Geometry check sheet. Reference: the model listing, model coordinates, mm. A direction names the side the tool comes from. Give positions to 0.01 mm unless a question says otherwise; leave off trailing zeros. Order: outer loops, then holes, each group sorted by start corner. A loop starts at its lowest first (then second) coordinate and runs counter-clockwise, first axis right, second up. Notation, with made-up numbers: M 76,-11.5 L 129,-11.5 A7 cw 129,-6.5 Z; hole C 85,11 d8. An arc over 180 degrees is marked long. Answer as CSV lines item,"result". Start each with the question number.
```python
from build123d import *

# Parameters (mm, degrees)
F0_R     = 6.35
F1_DEPTH = 16.002
F2_DEPTH = 16.002
F3_R     = 9.652
F4_W     = 56.33977
F4_H     = 23.11277
F5_DEPTH = 16.002
F7_R     = 9.652
F8_DEPTH = 16.003


with BuildPart() as f1:
    # F0 (on Front) → F1 (new body)
    with BuildSketch(Plane.XZ):
        with BuildLine():
            Line((-50.8, 0), (0, 0))
            Line((0, 0), (50.8, 0))
            Line((50.8, 0), (50.8, 44.45))
            ThreePointArc((50.8, 44.45), (47.080256, 53.430256), (38.1, 57.15))
            ThreePointArc((38.1, 57.15), (29.119744, 53.430256), (25.4, 44.45))
            Line((25.4, 44.45), (25.4, 16.002))
            Line((25.4, 16.002), (0, 16.002))
            Line((0, 16.002), (-25.4, 16.002))
            Line((-25.4, 16.002), (-25.4, 44.45))
            ThreePointArc((-25.4, 44.45), (-29.119744, 53.430256), (-38.1, 57.15))
            ThreePointArc((-38.1, 57.15), (-47.080256, 53.430256), (-50.8, 44.45))
            Line((-50.8, 44.45), (-50.8, 0))
        make_face()
        with Locations((-38.1, 44.45)):
            Circle(F0_R, mode=Mode.SUBTRACT)
        with Locations((38.1, 44.45)):
            Circle(F0_R, mode=Mode.SUBTRACT)
    extrude(amount=F1_DEPTH)

    # F0 (on Front) → F2 (join)
    with BuildSketch(Plane.XZ):
        with BuildLine():
            Line((-50.8, 0), (0, 0))
            Line((0, 0), (50.8, 0))
            Line((50.8, 0), (50.8, 44.45))
            ThreePointArc((50.8, 44.45), (47.080256, 53.430256), (38.1, 57.15))
            ThreePointArc((38.1, 57.15), (29.119744, 53.430256), (25.4, 44.45))
            Line((25.4, 44.45), (25.4, 16.002))
            Line((25.4, 16.002), (0, 16.002))
            Line((0, 16.002), (-25.4, 16.002))
            Line((-25.4, 16.002), (-25.4, 44.45))
            ThreePointArc((-25.4, 44.45), (-29.119744, 53.430256), (-38.1, 57.15))
            ThreePointArc((-38.1, 57.15), (-47.080256, 53.430256), (-50.8, 44.45))
            Line((-50.8, 44.45), (-50.8, 0))
        make_face()
        with Locations((-38.1, 44.45)):
            Circle(F0_R, mode=Mode.SUBTRACT)
        with Locations((38.1, 44.45)):
            Circle(F0_R, mode=Mode.SUBTRACT)
    extrude(amount=F2_DEPTH)

    # F3
    f3_edges = [f1.edges().sort_by_distance(p)[0] for p in [
        (-25.4, -8.001, 16.002),
        (25.4, -8.001, 16.002),
    ]]
    fillet(f3_edges, radius=F3_R)

    # F4 (on Top) → F5 (join)
    with BuildSketch(Plane.XY):
        with Locations((0, -27.554179)):
            Rectangle(F4_W, F4_H)
    extrude(amount=F5_DEPTH)

    # F7
    f7_edges = [f1.edges().sort_by_distance(p)[0] for p in [
        (28.169885, -39.110564, 8.001),
        (-28.169885, -39.110564, 8.001),
        (28.169885, -16.002, 8.001),
        (-28.169885, -16.002, 8.001),
    ]]
    fillet(f7_edges, radius=F7_R)

    # F6 (on face) → F8 (cut, through all)
    with BuildSketch(Plane.XY.offset(16.002)):
        with BuildLine():
            Line((19.05, -21.026887), (0, -21.026887))
            Line((0, -21.026887), (-19.05, -21.026887))
            ThreePointArc((-19.05, -21.026887), (-25.4, -27.376887), (-19.05, -33.726887))
            Line((-19.05, -33.726887), (0, -33.726887))
            Line((0, -33.726887), (19.05, -33.726887))
            ThreePointArc((19.05, -33.726887), (25.4, -27.376887), (19.05, -21.026887))
        make_face()
    extrude(amount=-F8_DEPTH, mode=Mode.SUBTRACT)


solid = f1.part
```
Item 1: Depth check by flat-ended pin: pin 1 Ø10.5 at (x, z) = (-27.5, 23.5) entering from -Y; pin 2 Ø5 at (y, z) = (-19.5, 16.5) entering from -X; pin 3 Ø4 at (y, z) = (-27.5, 11.5) entering from -X. Enter the tip coordinate at first touch or a pass-through.
Item 2: Draft check along X on faces 1 (the face through (0, -39.111, 8)), 2 (the face through (-1, -19, 16.002)), 3 (the face through (-30.922, -18.904, 7.889)). Enter one of: pulls with the +X half, pulls with the -X half, needs draft (parallel to the pull), parting line crosses it, or undercut.
Item 3: Section check A-A on z = 32. Record the boundary of the cut face in (x, y), then the cut area to 3 significant figures.
Item 4: Section check B-B on y = -9.5. Record the boundary of the cut face in (x, z).
Item 5: Scan lines: line 1 along X through (y, z) = (-9, 44); line 2 along Z through (x, y) = (38, -3); line 3 along X through (y, z) = (-1.5, 48.5). Record each from-to range of solid material in increasing order.
Item 6: Section check D-D on z = 49.5. Record the boundary of the cut face in (x, y).
Item 7: Access from +Z, -Z, +X, -X, +Y, -Y to the whole of each face (thin tool, end or side, straight path). Record for faces 4 (the face through (41, -16.002, 29)), 5 (the face through (25.4, -27.5, 8.1)), 6 (the face through (-25.4, -8, 35)), 7 (the face through (-28.17, -28, 8)).
Item 8: Section check C-C on x = -2.5. Record the boundary of the cut face in (y, z), then the cut area to 3 significant figures.
Numbers:
1,pin 1,"y = -16"
1,pin 2,"x = -33.45"
1,pin 3,"x = -28.17"
2,face 1,"needs draft"
2,face 2,"undercut"
2,face 3,"pulls with the -X half"
3,outline,"M -50.8,-16 L -25.4,-16 L -25.4,0 L -50.8,0 Z; M 25.4,-16 L 50.8,-16 L 50.8,0 L 25.4,0 Z"
3,area,"813 mm2"
4,outline,"M -50.8,0 L 50.8,0 L 50.8,44.45 A12.7 ccw 25.4,44.45 L 25.4,25.65 A9.65 cw 15.75,16 L -15.75,16 A9.65 cw -25.4,25.65 L -25.4,44.45 A12.7 ccw -50.8,44.45 Z; hole C -38.1,44.45 d12.7; hole C 38.1,44.45 d12.7"
5,line 1,"-50.8 to -44.43, -31.77 to -25.4, 25.4 to 31.77, 44.43 to 50.8"
5,line 2,"0 to 38.1, 50.8 to 57.15"
5,line 3,"-50.14 to -42.99, -33.21 to -26.06, 26.06 to 33.21, 42.99 to 50.14"
6,outline,"M -49.75,-16 L -41.95,-16 L -41.95,0 L -49.75,0 Z; M -34.25,-16 L -26.45,-16 L -26.45,0 L -34.25,0 Z; M 26.45,-16 L 34.25,-16 L 34.25,0 L 26.45,0 Z; M 41.95,-16 L 49.75,-16 L 49.75,0 L 41.95,0 Z"
7,face 4,"+Z, +X, -Y"
7,face 5,"+Z, -Z"
7,face 6,"+Z, +Y, -Y"
7,face 7,"+Z, -Z, -X, -Y"
8,outline,"M -39.11,0 L -33.73,0 L -33.73,16 L -39.11,16 Z; M -21.03,0 L 0,0 L 0,16 L -21.03,16 Z"
8,area,"423 mm2"
